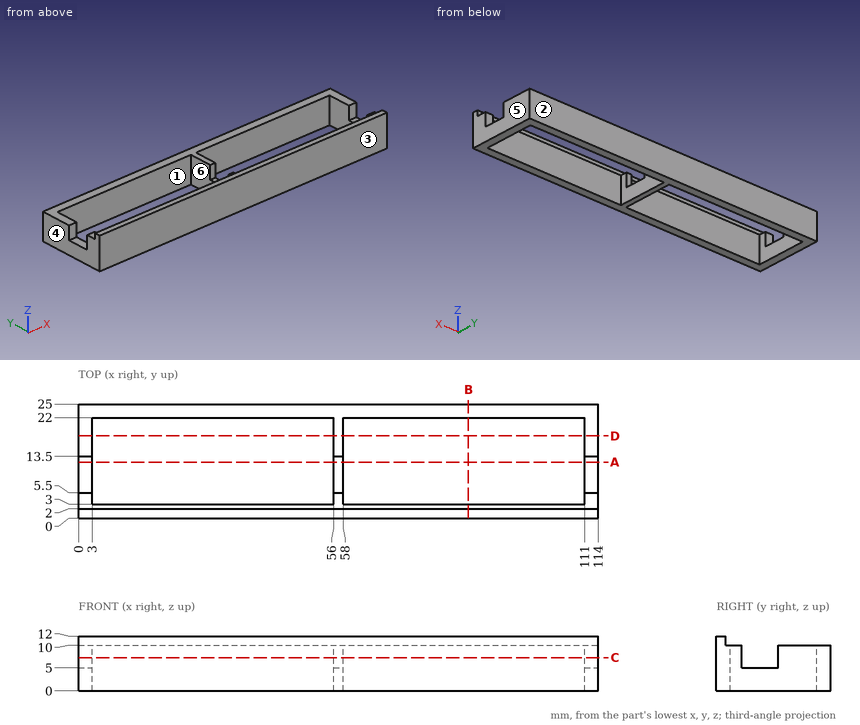
Check sheet for the drawn part. Datum: minimum x, y, z corner. Units: mm. A direction names the side the tool comes from. Coordinates: 2 decimals unless noted, no trailing zeros. Loops run counter-clockwise (first coordinate to the right, second up) from the corner with the lowest first, then second, coordinate; pieces in that order, holes last. Notation, with made-up numbers: (68, 77) -> (126, 77) arc R13 ccw to (126, 92) -> close; hole circle Ø5 at (56, 45.5). An arc over 180 degrees is marked (long way). Write each question's results on one line, items separated by ' | '.
Item 1: Section check B-B, the plane x = 85.5. Enter the section's corners in (y, z).
Found:
outline: (0, 0) -> (3, 0) -> (3, 10) -> (2, 10) -> (2, 12) -> (0, 12) -> close; (22, 0) -> (25, 0) -> (25, 10) -> (22, 10) -> close
Item 2: Tool access check on the marked faces 5 and 6. Record the directions out of +Z, -Z, +X, -X, +Y, -Y that give a thin tool (end or side, any length) a straight path to the whole face; none if there is none.
Found:
face 5: +Z, -Z, +X, +Y, -Y | face 6: +Z, -Z
Item 3: Section check C-C, the plane z = 7.25. Enter the section's corners in (x, y).
Found:
outline: (0, 0) -> (114, 0) -> (114, 5.5) -> (111, 5.5) -> (111, 3) -> (58, 3) -> (58, 5.5) -> (56, 5.5) -> (56, 3) -> (3, 3) -> (3, 5.5) -> (0, 5.5) -> close; (0, 13.5) -> (3, 13.5) -> (3, 22) -> (56, 22) -> (56, 13.5) -> (58, 13.5) -> (58, 22) -> (111, 22) -> (111, 13.5) -> (114, 13.5) -> (114, 25) -> (0, 25) -> close
Item 4: Material ranges on L1, parallel to X at y = 21, z = 5; L2, parallel to Y at x = 17, z = 1.5; L3, parallel to Y at x = 51, z = 10.75, recorded low to high.
Found:
L1: x = 0 to 3, 56 to 58, 111 to 114 | L2: y = 0 to 3, 22 to 25 | L3: y = 0 to 2
Item 5: Section check D-D, the plane y = 18. Enter the section's corners in (x, z), plus the area to 3 significant figures.
Found:
outline: (0, 0) -> (3, 0) -> (3, 10) -> (0, 10) -> close; (56, 0) -> (58, 0) -> (58, 10) -> (56, 10) -> close; (111, 0) -> (114, 0) -> (114, 10) -> (111, 10) -> close | area: 80.0 mm2
Item 6: Section check A-A, the plane y = 12.25. Enter the section's corners in (x, z), plus the area to 3 significant figures.
Found:
outline: (0, 0) -> (3, 0) -> (3, 5) -> (0, 5) -> close; (56, 0) -> (58, 0) -> (58, 5) -> (56, 5) -> close; (111, 0) -> (114, 0) -> (114, 5) -> (111, 5) -> close | area: 40.0 mm2
Item 7: Mould release check, pull along Y, two halves, no side actions. Record for the marked faces 1, 2, 3 and 4: +Y half, -Y half, draft (parallel to the pull), parting line (faces both ways), or undercut.
Found:
face 1: undercut | face 2: +Y half | face 3: -Y half | face 4: draft
Item 8: Gauge pin test, flat ends, axial feed: pin 1 (5 mm diameter, centred on x = 52.5, y = 22.5, fed in from -Z); pin 2 (2.5 mm diameter, centred on x = 113, y = 10, fed in from +Z); pin 3 (1 mm diameter, centred on x = 79.5, y = 3, fed in from +Z); pin 4 (1 mm diameter, centred on x = 33, z = 11.5, fed in from +Y). Record the tip position at first contact, or that the pin passes through.
Found:
pin 1: stops at z = 0 | pin 2: stops at z = 5 | pin 3: stops at z = 10 | pin 4: stops at y = 2
